The model under review builds one solid part; all positions refer to its coordinate system, in mm. A direction names the side the tool comes from. Give positions to 0.01 mm unless a question says otherwise; leave off trailing zeros. Loops run counter-clockwise (first coordinate to the right, second up) from the corner with the lowest first, then second, coordinate; pieces in that order, holes last. Notation, with made-up numbers: (14, -8) - (28, -8) arc R26 ccw to (28, 15) - close; hole circle Ø6 at (60.5, -8.5). An arc over 180 degrees is marked (long way). Answer as a JSON object with one key per item and string values.
from build123d import *

# Parameters (mm, degrees)
F0_R     = 1.6
F1_DEPTH = 1
F2_R     = 1.5
F3_W     = 140
F3_H     = 1
F4_DEPTH = 6
F5_W     = 63.5
F5_H     = 1.5
F5_W_2   = 1.5
F5_H_2   = 93.5
F6_DEPTH = 1.5
F7_R     = 1.4999
F8_W     = 10
F8_H     = 2
F9_DEPTH = 1.5


# Not quite as in the source:
# - a fillet or chamfer is up to 0.001 mm smaller than in the source, because OpenCascade refuses the exact size


with BuildPart() as f1:
    # F0 (on Top) → F1 (new body)
    with BuildSketch(Plane.XY):
        Polygon((69.4188682817, 0), (-37.5811317183, 0), (-37.5811317183, -10), (69.4188682817, -10), (69.4188682817, -30), (134.4188682817, -30), (134.4188682817, -10), (155.4188682817, -10), (155.4188682817, 0), (134.4188682817, 0), (134.4188682817, 65), (69.4188682817, 65), align=None)
        with Locations((-30.9811317183, -5)):
            Circle(F0_R, mode=Mode.SUBTRACT)
        with Locations((150.0188682817, -5)):
            Circle(F0_R, mode=Mode.SUBTRACT)
    extrude(amount=F1_DEPTH)

    # F2
    f2_edges = [f1.edges().sort_by_distance(p)[0] for p in [
        (-37.581132, 0, 0.5),
        (-37.581132, -10, 0.5),
        (155.418868, 0, 0.5),
        (155.418868, -10, 0.5),
        (134.418868, -30, 0.5),
        (69.418868, -30, 0.5),
        (69.418868, 65, 0.5),
        (134.418868, 65, 0.5),
    ]]
    fillet(f2_edges, radius=F2_R)

    # F3 (on face) → F4 (join)
    with BuildSketch(Plane(origin=(0, 0, 0), x_dir=(1, 0, 0), z_dir=(0, 0, -1))):
        with Locations((62.4188682817, 5)):
            Rectangle(F3_W, F3_H)
    extrude(amount=F4_DEPTH)

    # F5 (on face) → F6 (join)
    with BuildSketch(Plane.XY.offset(1)):
        with Locations((101.1688682817, -29.25)):
            Rectangle(F5_W, F5_H)
        with Locations((133.6688682817, 18.25)):
            Rectangle(F5_W_2, F5_H_2)
        with Locations((133.6688682817, -29.25)):
            Rectangle(F5_W_2, F5_H)
    extrude(amount=F6_DEPTH)

    # F7 (radius 1.5 in the source; OpenCascade refuses exactly that, so slightly less here)
    f7_edges = [f1.edges().sort_by_distance(p)[0] for p in [
        (134.418868, -30, 1.75),
        (69.418868, -30, 1.75),
        (134.418868, 65, 1.75),
    ]]
    fillet(f7_edges, radius=F7_R)

    # F8 (on face) → F9 (join, through all)
    with BuildSketch(Plane.XY.offset(1)):
        with Locations((139.4188682817, -5)):
            Rectangle(F8_W, F8_H)
    extrude(amount=F9_DEPTH)


solid = f1.part
Q1. Consider section C-C, the plane z = -2.75. State the section outline as (x, y) points.
Results:
{"outline": "(-7.58, -5.5) - (132.42, -5.5) - (132.42, -4.5) - (-7.58, -4.5) - close"}
Q2. For faces 1 (the face through (61, -5.5, -3)), 2 (the face through (61, -4.5, -3)), 3 (the face through (84, 19, 1)), list the 3-axis set-ups (+Z, -Z, +X, -X, +Y, -Y) from which the entire face can be reached by the end or side of a thin tool; tool diameter is ignored.
Results:
{"face 1": "-Z, +X, -X, -Y", "face 2": "-Z, +X, -X, +Y", "face 3": "+Z, -X, +Y"}
Q3. Clearance check with flat-ended pins moving along their axes: pin 1 Ø0.8 at (y, z) = (41, 1.5) entering from -X; pin 2 Ø1 at (x, z) = (87, -1) entering from -Y; pin 3 Ø0.8 at (x, z) = (23.5, 0.5) entering from +Y. State where each tip first meets the part, or that it passes through.
Results:
{"pin 1": "stops at x = 132.92", "pin 2": "stops at y = -5.5", "pin 3": "stops at y = 0"}
Q4. Consider section D-D, the plane x = -17.5. State the section outline as (y, z) points.
Results:
{"outline": "(-10, 0) - (0, 0) - (0, 1) - (-10, 1) - close"}
Q5. Consider section A-A, the plane x = 117. State the section outline as (y, z) points, plus the area to 3 significant figures.
Results:
{"outline": "(-30, 0) - (-5.5, 0) - (-5.5, -6) - (-4.5, -6) - (-4.5, 0) - (65, 0) - (65, 1) - (-28.5, 1) - (-28.5, 2.5) - (-30, 2.5) - close", "area": "103 mm^2"}
Q6. Consider section B-B, the plane y = 13. State the section outline as (x, z) points.
Results:
{"outline": "(69.42, 0) - (134.42, 0) - (134.42, 2.5) - (132.92, 2.5) - (132.92, 1) - (69.42, 1) - close"}
Q7. To check wall thickness, follow probe 1 along Y at (x, z) = (119.5, -3.5); probe 2 along Z at (x, y) = (125.5, 60.5); probe 3 along X at (y, z) = (8.5, 0.75). State the ranges of each line that lie inside material, in increasing order. Write a range as [from, to].
Results:
{"probe 1": "y = [-5.5, -4.5]", "probe 2": "z = [0, 1]", "probe 3": "x = [69.42, 134.42]"}
